from build123d import *

# Parameters (mm, degrees)
EXTRUSION1_DEPTH = 3
EXTRUSION2_DEPTH = 4


with BuildPart() as part:
    # Esquisse1 → Extrusion1 (new body)
    with BuildSketch(Plane.XY):
        with BuildLine():
            Line((-5, 8.660254038), (-5, 40))
            ThreePointArc((-5, 40), (0, 45), (5, 40))
            Line((5, 40), (5, 8.660254038))
            ThreePointArc((5, 8.660254038), (0, -10), (-5, 8.660254038))
        make_face()
    extrude(amount=EXTRUSION1_DEPTH)

    # Esquisse2 → Extrusion2 (cut, through all)
    with BuildSketch(Plane.XY.offset(3)):
        with BuildLine():
            Line((-1.936491673, 3.5), (1.936491673, 3.5))
            ThreePointArc((1.936491673, 3.5), (0, -4), (-1.936491673, 3.5))
        make_face()
    extrude(amount=-EXTRUSION2_DEPTH, mode=Mode.SUBTRACT)


solid = part.part
Input: part model. Units: mm. Frame: model coordinates. A direction names the side the tool comes from. Round coordinates to 2 decimals unless told otherwise and drop trailing zeros. Write each loop counter-clockwise with the first axis right and the second up, starting at its lowest first coordinate (ties: lowest second). Pieces come first, ordered by that corner, then holes.
1) Draft query along Y for faces 5 (the cylindrical face through (0, 45, 1)), 6 (the cylindrical face through (0, -4, 2)), 7 (the flat face through (0, 18, 3)). Return one class per face: pulls with the +Y half, pulls with the -Y half, needs draft (parallel to the pull), parting line crosses it, or undercut.
2) Contact query for flat-ended pins moving along their axis: P1, Ø8, axis at x = -7, y = 32.5, coming from the -Z side; P2, Ø1, axis at x = -1, z = 0.5, coming from the +Y side; P3, Ø6.5, axis at x = 0, y = 0, coming from the -Z side; P4, Ø1.5, axis at x = 4, z = 1.5, coming from the -Y side. Output: stop coordinate, or through.
3) Cut plane C-C (z = 1.3). Return the cut outline in (x, y), then the cut area to 3 significant figures.
4) Cut plane A-A (x = 0). Return the cut outline in (y, z), then the cut area to 4 significant figures.
5) Ray query, L1, parallel to Y at x = 0, z = 1.75; L2, parallel to X at y = 13, z = 2.75; L3, parallel to Y at x = -3.25, z = 0.65. Return the intervals inside material, ascending.
6) Cut plane B-B (y = 0). Return the cut outline in (x, z), then the cut area to 3 significant figures.
7) Cut plane D-D (y = 30.5). Return the cut outline in (x, z).
8) Reachability of faces 1 (the flat face through (0, 18, 0)), 2 (the flat face through (-5, 24, 1)), 3 (the flat face through (5, 25, 1)), 4 (the flat face through (0, 3.5, 2)) from +Z, -Z, +X, -X, +Y, -Y: full face, straight path, thin tool, end or side. Return the list, or none.
Geometry says:
1. face 5: pulls with the +Y half
1. face 6: undercut
1. face 7: needs draft
2. P1: stops at z = 0
2. P2: stops at y = 44.97
2. P3: passes through
2. P4: stops at y = -9.46
3. outline: (-5, 8.66) arc R10 ccw (long way) to (5, 8.66) - (5, 40) arc R5 ccw to (-5, 40) - close; hole (-1.94, 3.5) arc R4 ccw (long way) to (1.94, 3.5) - close
3. area: 609 mm2
4. outline: (-10, 0) - (-4, 0) - (-4, 3) - (-10, 3) - close; (3.5, 0) - (45, 0) - (45, 3) - (3.5, 3) - close
4. area: 142.5 mm2
5. L1: y = -10 to -4, 3.5 to 45
5. L2: x = -5 to 5
5. L3: y = -9.46 to -2.33, 2.33 to 43.8
6. outline: (-10, 0) - (-4, 0) - (-4, 3) - (-10, 3) - close; (4, 0) - (10, 0) - (10, 3) - (4, 3) - close
6. area: 36.0 mm2
7. outline: (-5, 0) - (5, 0) - (5, 3) - (-5, 3) - close
8. face 1: -Z, +X, -X, +Y, -Y
8. face 2: +Z, -Z, -X, +Y
8. face 3: +Z, -Z, +X, +Y
8. face 4: +Z, -Z
